CAD build for the part. Positions are in the model's coordinates, mm. A direction names the side the tool comes from. Round coordinates to 2 decimals unless told otherwise and drop trailing zeros. Order: outer loops, then holes, each group sorted by start corner. A loop starts at its lowest first (then second) coordinate and runs counter-clockwise, first axis right, second up. Notation, with made-up numbers: M 1.25,-32 L 31.25,-32 A34 ccw 31.25,3 Z; hole C 36,71.5 d5. An arc over 180 degrees is marked long. Answer as a JSON object with one key per item and string values.
```python
from build123d import *

# Parameters (mm, degrees)
EXTRUDE_1_DEPTH = 20
FILLET_1_R      = 20


with BuildPart() as part:
    # 草圖1 → 填料-伸長1 (new body)
    with BuildSketch(Plane.XY):
        Polygon((0, 179.483059357), (-185, -140.946340043), (185, -140.946340043), align=None)
        Polygon((0, 139.483059357), (-150.358983849, -120.946340043), (150.358983849, -120.946340043), align=None, mode=Mode.SUBTRACT)
    extrude(amount=EXTRUDE_1_DEPTH)

    # 圓角1
    fillet_1_edges = [part.edges().sort_by_distance(p)[0] for p in [
        (185, -140.946340043, 10),
        (-185, -140.946340043, 10),
        (0, 179.483059357, 10),
    ]]
    fillet(fillet_1_edges, radius=FILLET_1_R)


solid = part.part
```
Item 1: Saw through at B-B on x = -105. List the corners of the cut face in (y, z), and give its area (3 significant figures).
Worked answers:
{"outline": "M -140.95,0 L -120.95,0 L -120.95,20 L -140.95,20 Z; M -42.38,0 L -2.38,0 L -2.38,20 L -42.38,20 Z", "area": "1,200 mm2"}
Item 2: Saw through at A-A on z = 17. List the corners of the cut face in (x, y), and give its area (3 significant figures).
Worked answers:
{"outline": "M -167.68,-110.95 A20 ccw -150.36,-140.95 L 150.36,-140.95 A20 ccw 167.68,-110.95 L 17.32,149.48 A20 ccw -17.32,149.48 Z; hole M -150.36,-120.95 L 150.36,-120.95 L 0,139.48 Z", "area": "19,300 mm2"}
Item 3: Wall check: line 1 along Y through (x, z) = (57, 3.5); line 2 along Y through (x, z) = (-68.5, 18.25); line 3 along X through (y, z) = (119, 13.5). Give the ranges that are in metal, low to high. Write a range as [from, to].
Worked answers:
{"line 1": "y = [-140.95, -120.95], [40.76, 80.76]", "line 2": "y = [-140.95, -120.95], [20.84, 60.84]", "line 3": "x = [-34.92, -11.83], [11.83, 34.92]"}
Item 4: 3-axis set-ups, long thin cutter, end or side, ignore diameter. For faces 4 (the flat face through (-91.45, 21.09, 9.86)), 5 (the flat face through (-2, -120.946, 10)): which of +Z, -Z, +X, -X, +Y, -Y reach the whole face in a straight line?
Worked answers:
{"face 4": "+Z, -Z, -X, +Y", "face 5": "+Z, -Z"}
Item 5: Two-plate mould, pull along Y, no slides. Class faces 1 (the flat face through (-2, -140.946, 10)), 2 (the flat face through (76.23, 7.45, 9.86)), 3 (the flat face through (-77, 10, 20)): released by +Y, released by -Y, zero draft, split by the parting line, or undercut.
Worked answers:
{"face 1": "released by -Y", "face 2": "undercut", "face 3": "zero draft"}
Item 6: Saw through at C-C on y = -68.5. List the corners of the cut face in (x, z).
Worked answers:
{"outline": "M -143.17,0 L -120.08,0 L -120.08,20 L -143.17,20 Z; M 120.08,0 L 143.17,0 L 143.17,20 L 120.08,20 Z"}
Item 7: Drop flat-ended pins along their axis: pin 1 Ø12 at (x, z) = (-8.5, 2.5) entering from +Y; pin 2 Ø8 at (y, z) = (-5, 14) entering from -X; pin 3 Ø1 at (y, z) = (-39.5, 8) entering from +X. Give the stop position or say it passes through.
Worked answers:
{"pin 1": "stops at y = 159.33", "pin 2": "stops at x = -108.82", "pin 3": "stops at x = 126.72"}
